Source: three-view drawing plus pictorial views. Frame: mm from the lowest corner of the part. Give positions to 0.01 mm unless a question says otherwise; leave off trailing zeros. Loops run counter-clockwise (first coordinate to the right, second up) from the corner with the lowest first, then second, coordinate; pieces in that order, holes last. Notation, with made-up numbers: M 49.25,35.25 L 66.25,35.25 A29 ccw 66.25,62.25 Z; hole C 75,3.5 d2. An arc over 180 degrees is marked long. Answer as a JSON object with one key per item and string values. Group by question number.
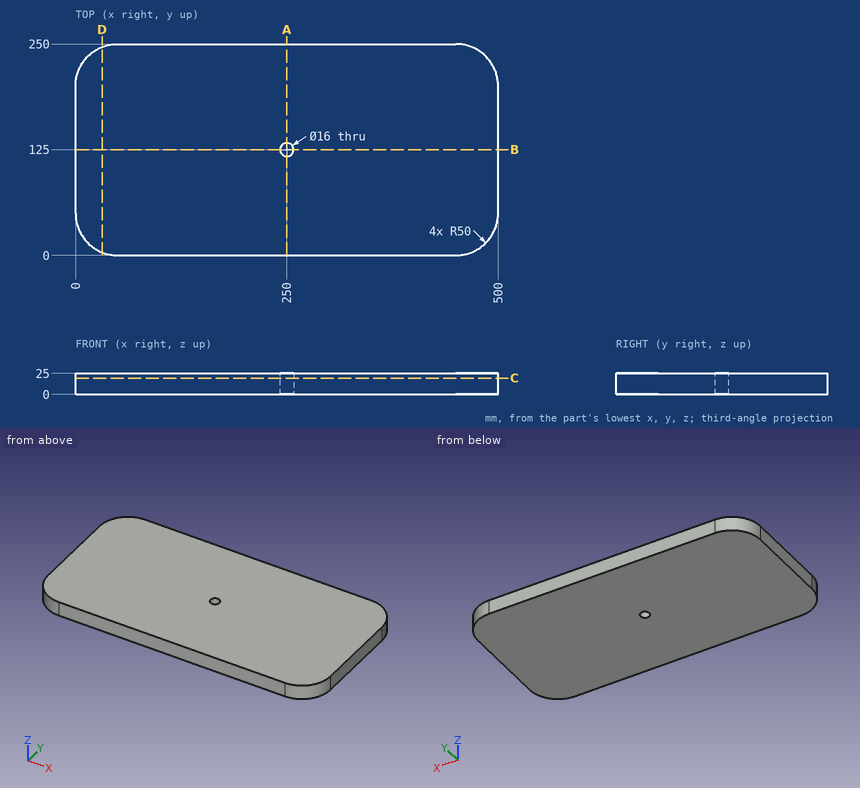
1. Section B-B (y = 125). Output: boundary loops of the cut face in (x, z).
2. Section A-A (x = 250). Output: boundary loops of the cut face in (y, z), then the cut area to 3 significant figures.
3. Material intervals for L1, parallel to Y at x = 250, z = 7; L2, parallel to Y at x = 461, z = 10.25 (3 decimals); L3, parallel to X at y = 213, z = 13.75, sorted ascending.
4. First-contact query: P1, Ø1.5, axis at y = 29.5, z = 19, coming from the -X side. Flat tip, straight axial feed; report the tip coordinate or a pass-through.
5. Section D-D (x = 31.5). Output: boundary loops of the cut face in (y, z), then the cut area to 3 significant figures.
6. Section C-C (z = 19.25). Output: boundary loops of the cut face in (x, y), then the cut area to 3 significant figures.
Geometry results:
{
 "1": {"outline": "M 0,0 L 242,0 L 242,25 L 0,25 Z; M 258,0 L 500,0 L 500,25 L 258,25 Z"},
 "2": {"outline": "M 0,0 L 117,0 L 117,25 L 0,25 Z; M 133,0 L 250,0 L 250,25 L 133,25 Z", "area": "5,850 mm2"},
 "3": {"L1": "0 to 117, 133 to 250", "L2": "1.225 to 248.775", "L3": "1.72 to 498.28"},
 "4": {"P1": "x = 4.07"},
 "5": {"outline": "M 3.55,0 L 246.45,0 L 246.45,25 L 3.55,25 Z", "area": "6,070 mm2"},
 "6": {"outline": "M 0,50 A50 ccw 50,0 L 450,0 A50 ccw 500,50 L 500,200 A50 ccw 450,250 L 50,250 A50 ccw 0,200 Z; hole C 250,125 d16", "area": "123,000 mm2"}
}
